For this review, use the dimensioned drawing (mm, ordinates from the lowest corner) and the shaded views. Coordinates: 2 decimals unless noted, no trailing zeros. Loops run counter-clockwise (first coordinate to the right, second up) from the corner with the lowest first, then second, coordinate; pieces in that order, holes last.
1. Take a section at A-A, the plane z = 44.5. State the section outline as (x, y) points.
2. Take a section at D-D, the plane z = 32. State the section outline as (x, y) points (1 decimal).
3. To check wall thickness, follow probe 1 along Z at (x, y) = (11, 0.55) (1 decimal); probe 2 along X at (y, z) = (0.7, 78) (1 decimal); probe 3 along Z at (x, y) = (12, 0.2) (1 decimal). State the ranges of each line that lie inside material, in increasing order.
4. Take a section at C-C, the plane x = 62. State the section outline as (y, z) points, then the cut area to 3 significant figures.
5. Take a section at B-B, the plane y = 1.3. Count the separate pieces of the cut face and the enclosed holes in it, then the cut area to 3 significant figures.
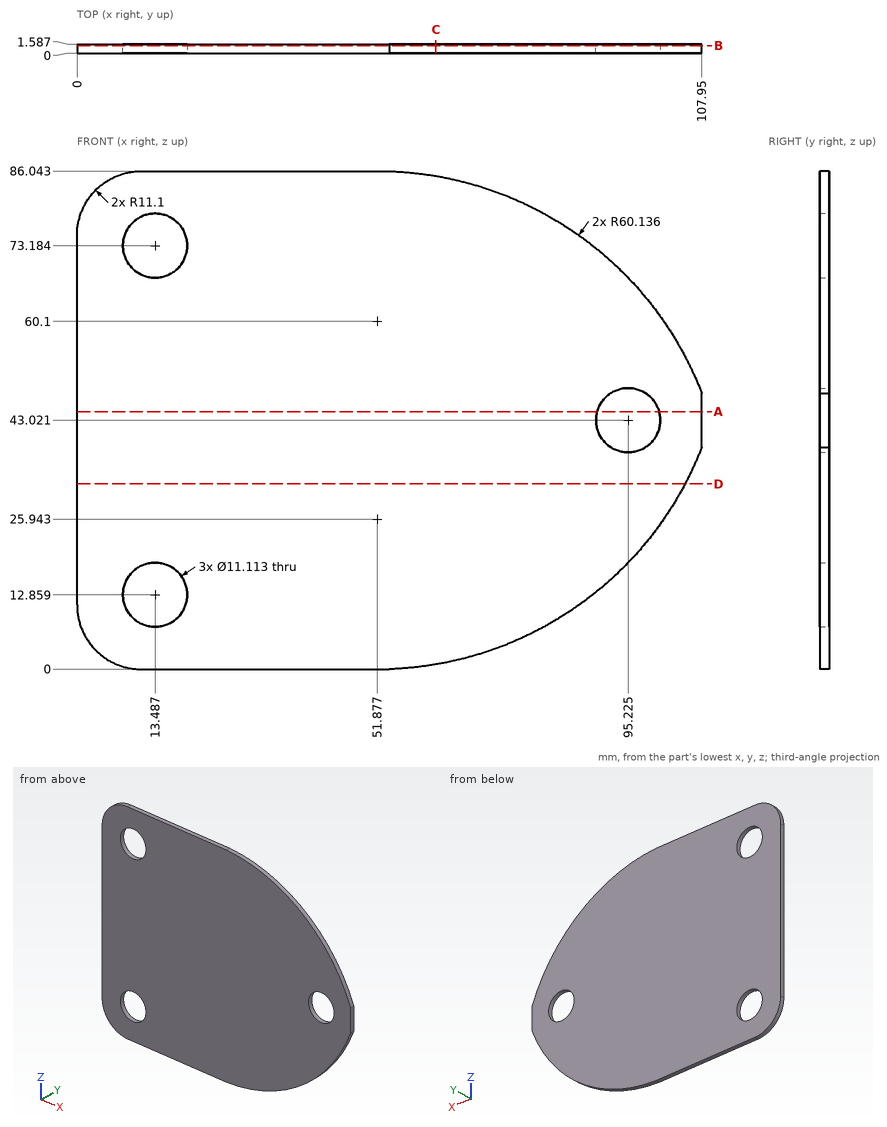
Results list:
1. outline: (0, 0) - (89.87, 0) - (89.87, 1.59) - (0, 1.59) - close; (100.58, 0) - (107.95, 0) - (107.95, 1.59) - (100.58, 1.59) - close
2. outline: (0, 0) - (105, 0) - (105, 1.6) - (0, 1.6) - close
3. probe 1: z = 0 to 7.9, 17.8 to 68.2, 78.2 to 86
3. probe 2: x = 0.4 to 10.7, 16.3 to 82
3. probe 3: z = 0 to 7.5, 18.2 to 67.8, 78.5 to 86
4. outline: (0, 0.82) - (1.59, 0.82) - (1.59, 85.22) - (0, 85.22) - close
4. area: 134 mm2
5. separate pieces: 1
5. enclosed holes: 3
5. area: 7,770 mm2
